from build123d import *

# Parameters (mm, degrees)
SKETCH1_W           = 40
SKETCH1_H           = 20
BOSS_EXTRUDE1_DEPTH = 2
SKETCH2_W           = 40
SKETCH2_H           = 2
BOSS_EXTRUDE2_DEPTH = 20
SKETCH3_R           = 1.75
CUT_EXTRUDE1_DEPTH  = 23
SKETCH4_R           = 5
SKETCH4_R_2         = 1
CUT_EXTRUDE2_DEPTH  = 21


with BuildPart() as part:
    # Sketch1 → Boss-Extrude1 (new body)
    with BuildSketch(Plane(origin=(0, 0, 0), x_dir=(1, 0, 0), z_dir=(0, 1, 0))):
        Rectangle(SKETCH1_W, SKETCH1_H)
    extrude(amount=BOSS_EXTRUDE1_DEPTH)

    # Sketch2 → Boss-Extrude2 (add)
    with BuildSketch(Plane(origin=(0, 2, 0), x_dir=(1, 0, 0), z_dir=(0, 1, 0))):
        with Locations((0, 9)):
            Rectangle(SKETCH2_W, SKETCH2_H)
    extrude(amount=BOSS_EXTRUDE2_DEPTH)

    # Sketch3 → Cut-Extrude1 (cut, through all)
    with BuildSketch(Plane.XZ):
        with Locations((-14, 2)):
            Circle(SKETCH3_R)
        with Locations((14, 2)):
            Circle(SKETCH3_R)
    extrude(amount=-CUT_EXTRUDE1_DEPTH, mode=Mode.SUBTRACT)

    # Sketch4 → Cut-Extrude2 (cut, through all)
    with BuildSketch(Plane(origin=(0, 0, -10), x_dir=(-1, 0, 0), z_dir=(0, 0, -1))):
        with Locations((0, 13.5)):
            Circle(SKETCH4_R)
        with Locations((-9.5, 16.5)):
            Circle(SKETCH4_R_2)
        with Locations((9.5, 16.5)):
            Circle(SKETCH4_R_2)
    extrude(amount=-CUT_EXTRUDE2_DEPTH, mode=Mode.SUBTRACT)


solid = part.part
For this review, take the finished solid that the model builds, in its own axes (mm). A direction names the side the tool comes from. Round coordinates to 2 decimals unless told otherwise and drop trailing zeros. Loops run counter-clockwise (first coordinate to the right, second up) from the corner with the lowest first, then second, coordinate; pieces in that order, holes last. Notation, with made-up numbers: (42, 83.5) - (85, 83.5) arc R35 cw to (85, 121.5) - close; hole circle Ø9 at (52, 36). An arc over 180 degrees is marked (long way). Use one line per item in the form item = value.
1) Mouldability with a two-part tool opening along Y and no side actions: class faces 3 (the face through (0, 22, -9)), 4 (the face through (4, 10.5, -9)), 5 (the face through (0, 0, 0)) as pulls with the +Y half, pulls with the -Y half, needs draft (parallel to the pull), parting line crosses it, or undercut.
Solutions:
face_3 = pulls with the +Y half
face_4 = undercut
face_5 = pulls with the -Y half
2) Tool access review of faces 1 (the face through (0, 1, 10)), 2 (the face through (0, 2, 1)): name each direction out of +Z, -Z, +X, -X, +Y, -Y from which nothing blocks a thin tool from reaching the whole face with its end or side.
Solutions:
face_1 = +Z, +X, -X, +Y, -Y
face_2 = +Z, +X, -X, +Y
3) Clearance check with flat-ended pins moving along their axes: P1, Ø4, axis at x = 14, z = 2, coming from the +Y side; P2, Ø1.6, axis at x = 9.5, y = 16.5, coming from the +Z side; P3, Ø4, axis at x = -3, y = 18, coming from the +Z side. State where each tip first meets the part, or that it passes through.
Solutions:
P1 = 2
P2 = through
P3 = -8
4) Wall thickness on probe 1 along Z at (x, y) = (14, 1.2); probe 2 along Y at (x, z) = (0, -8.65); probe 3 along Y at (x, z) = (-9.5, -8.85): over which ranges is each line inside the solid? List them lowest first.
Solutions:
probe_1 = -10 to 0.25, 3.75 to 10
probe_2 = 0 to 8.5, 18.5 to 22
probe_3 = 0 to 15.5, 17.5 to 22
5) We need section A-A on x = 9.5. Write out the cut boundary in (y, z), then the cut area to 3 significant figures.
Solutions:
outline = (0, -10) - (15.5, -10) - (15.5, -8) - (2, -8) - (2, 10) - (0, 10) - close; (17.5, -10) - (22, -10) - (22, -8) - (17.5, -8) - close
area = 76.0 mm2
6) We need section D-D on z = 2. Write out the cut boundary in (x, y), then the cut area to 3 significant figures.
Solutions:
outline = (-20, 0) - (-15.75, 0) - (-15.75, 2) - (-20, 2) - close; (-12.25, 0) - (12.25, 0) - (12.25, 2) - (-12.25, 2) - close; (15.75, 0) - (20, 0) - (20, 2) - (15.75, 2) - close
area = 66.0 mm2
7) We need section B-B on y = 13.5. Write out the cut boundary in (x, z).
Solutions:
outline = (-20, -10) - (-5, -10) - (-5, -8) - (-20, -8) - close; (5, -10) - (20, -10) - (20, -8) - (5, -8) - close
8) We need section C-C on z = -8.5. Write out the cut boundary in (x, y).
Solutions:
outline = (-20, 0) - (20, 0) - (20, 22) - (-20, 22) - close; hole circle Ø2 at (-9.5, 16.5); hole circle Ø10 at (0, 13.5); hole circle Ø2 at (9.5, 16.5)
